Source: CAD feature listing. Evaluate the final solid. Frame: model axes, mm. Face numbers are marked on the shaded views. Round coordinates to 2 decimals unless told otherwise and drop trailing zeros. Loops run counter-clockwise (first coordinate to the right, second up) from the corner with the lowest first, then second, coordinate; pieces in that order, holes last. Notation, with made-up numbers: (47, 48) -> (62, 48) arc R20 cw to (62, 55) -> close; hole circle Ø4 at (81.5, 52). An arc over 180 degrees is marked (long way). Return JSON: item names as keys, results as strings. Group by question number.
```python
from build123d import *

# Parameters (mm, degrees)
F3_D           = 4.699
F3_CSINK_D     = 7.7978
F3_CSINK_ANGLE = 82
F4_R           = 3.81
F5_SIZE2       = 5.08
F5_SIZE        = 2.54


with BuildPart() as f1:
    # F0 (on Front) → F1 (revolve)
    with BuildSketch(Plane.XZ):
        Polygon((-41.529, 0), (-11.049, 0), (-11.049, 50.8), (-16.129, 50.8), (-19.2372467909, 6.35), (-41.529, 6.35), align=None)
    revolve(axis=Axis((0, 0, 5.6630113419), (0, 0, 1)))

    # F3 (through all)
    with Locations(Plane.XY.offset(6.35)):
        with Locations((-30.48, 0), (0, 30.48), (30.48, 0), (0, -30.48)):
            CounterSinkHole(F3_D / 2, F3_CSINK_D / 2, counter_sink_angle=F3_CSINK_ANGLE)

    # F4
    f4_edges = [f1.edges().sort_by_distance(p)[0] for p in [
        (41.529, 0, 6.35),
        (19.237247, 0, 6.35),
    ]]
    fillet(f4_edges, radius=F4_R)

    # F5
    f5_edges = [f1.edges().sort_by_distance(p)[0] for p in [
        (11.049, 0, 0),
        (11.049, 0, 50.8),
        (-11.049, 0, 25.4),
    ]]
    chamfer(f5_edges, length=F5_SIZE, length2=F5_SIZE2)


solid = f1.part
```
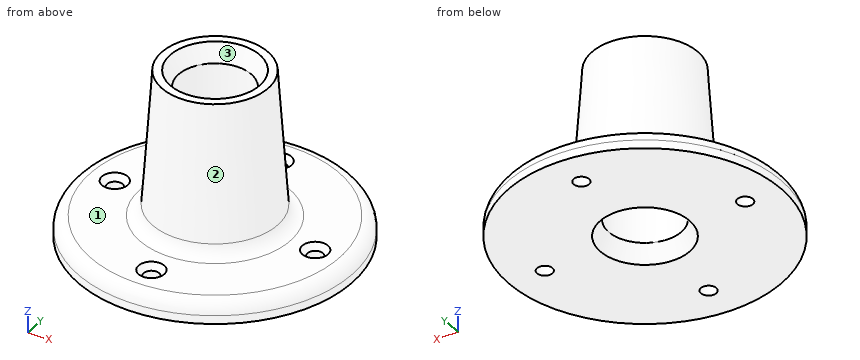
(1) Cut plane C-C (z = 42). Return loops of the section in (x, y).
(2) Cut plane A-A (x = 0). Count the separate pieces of the cut face and the enclosed holes in it, and give its area (3 significant figures).
(3) Mould query, pull axis X, two halves, no side actions, for the marked faces 1, 2 and 3. Classes: released by +X, released by -X, zero draft, split by the parting line, or undercut.
(4) Cut plane B-B (z = 34). Return loops of the section in (x, y), and give its area (3 significant figures).
(5) Ray query, line 1 (X direction, y = 0, z = 3.35); line 2 (Y direction, x = -30.48, z = 3.15); line 3 (Y direction, x = -30, z = 2). Return the intervals inside material, ascending.
(6) Pin query (flat end, axial travel): pin 1 (8 mm diameter, centred on x = 7.5, z = 44.5, fed in from -Y); pin 2 (8 mm diameter, centred on x = -18, z = 36, fed in from -Y); pin 3 (1 mm diameter, centred on x = -19, z = 29.5, fed in from -Y); pin 4 (10 mm diameter, centred on y = 6, z = 39, fed in from +X). Return the tip coordinate at first contact, or that it passes through.
Answers follow:
{
 "1": {"outline": "circle Ø33.49 at (0, 0); hole circle Ø22.1 at (0, 0)"},
 "2": {"separate pieces": "4", "enclosed holes": "0", "area": "885 mm^2"},
 "3": {"face 1": "zero draft", "face 2": "split by the parting line", "face 3": "undercut"},
 "4": {"outline": "circle Ø34.61 at (0, 0); hole circle Ø22.1 at (0, 0)", "area": "557 mm^2"},
 "5": {"line 1": "-41.44 to -32.83, -28.13 to -11.91, 11.91 to 28.13, 32.83 to 41.44", "line 2": "-28.13 to -2.35, 2.35 to 28.13", "line 3": "-28.72 to -2.3, 2.3 to 28.72"},
 "6": {"pin 1": "y = -16.24", "pin 2": "y = -9.95", "pin 3": "through", "pin 4": "x = 17.05"}
}
